from build123d import *

# Parameters (mm, degrees)
SKETCH_1_R      = 1.5
SKETCH_1_R_2    = 6.5
SKETCH_1_W      = 4
SKETCH_1_H      = 4.8
SKETCH_1_H_2    = 5
EXTRUDE_1_DEPTH = 4


with BuildPart() as part:
    # 草图1 → 凸台-拉伸1 (new body)
    with BuildSketch(Plane.XY):
        with BuildLine():
            Line((-11.37741807, 44.104762576), (9.62258193, 44.104762576))
            Line((9.62258193, 44.104762576), (17.62258193, 44.104762576))
            Line((17.62258193, 44.104762576), (38.62258193, 44.104762576))
            ThreePointArc((38.62258193, 44.104762576), (58.62258193, 24.104762576), (38.62258193, 4.104762576))
            Line((38.62258193, 4.104762576), (-11.37741807, 4.104762576))
            ThreePointArc((-11.37741807, 4.104762576), (-31.37741807, 24.104762576), (-11.37741807, 44.104762576))
        make_face()
        with Locations((1.12258193, 12.583043954)):
            Circle(SKETCH_1_R, mode=Mode.SUBTRACT)
        with Locations(Location((26.12258193, 12.583043954, 0), (0, 0, 180))):
            Circle(SKETCH_1_R, mode=Mode.SUBTRACT)
        with Locations((13.62258193, 24.104762576)):
            Circle(SKETCH_1_R, mode=Mode.SUBTRACT)
        with Locations((-11.37741807, 24.104762576)):
            Circle(SKETCH_1_R_2, mode=Mode.SUBTRACT)
        with Locations((38.62258193, 24.104762576)):
            Circle(SKETCH_1_R_2, mode=Mode.SUBTRACT)
        with Locations((29.363598717, 38.36208455)):
            Circle(SKETCH_1_R, mode=Mode.SUBTRACT)
        with Locations((-2.118434858, 38.36208455)):
            Circle(SKETCH_1_R, mode=Mode.SUBTRACT)
        with Locations((21.62258193, 37.474762576)):
            Rectangle(SKETCH_1_W, SKETCH_1_H, mode=Mode.SUBTRACT)
        with Locations((21.62258193, 28.344762576)):
            Rectangle(SKETCH_1_W, SKETCH_1_H_2, mode=Mode.SUBTRACT)
        with Locations((5.62258193, 37.474762576)):
            Rectangle(SKETCH_1_W, SKETCH_1_H, mode=Mode.SUBTRACT)
        with Locations((5.62258193, 28.344762576)):
            Rectangle(SKETCH_1_W, SKETCH_1_H_2, mode=Mode.SUBTRACT)
        with Locations((5.62258193, 19.114762576)):
            Rectangle(SKETCH_1_W, SKETCH_1_H_2, mode=Mode.SUBTRACT)
        with Locations((21.62258193, 19.114762576)):
            Rectangle(SKETCH_1_W, SKETCH_1_H_2, mode=Mode.SUBTRACT)
        with BuildLine():
            Line((11.87258193, 8.127075217), (11.87258193, 13.127075217))
            ThreePointArc((11.87258193, 13.127075217), (13.62258193, 14.877075217), (15.37258193, 13.127075217))
            Line((15.37258193, 13.127075217), (15.37258193, 8.127075217))
            ThreePointArc((15.37258193, 8.127075217), (13.62258193, 6.377075217), (11.87258193, 8.127075217))
        make_face(mode=Mode.SUBTRACT)
        with BuildLine():
            Line((15.37258193, 40.127075217), (15.37258193, 35.127075217))
            ThreePointArc((15.37258193, 35.127075217), (13.62258193, 33.377075217), (11.87258193, 35.127075217))
            Line((11.87258193, 35.127075217), (11.87258193, 40.127075217))
            ThreePointArc((11.87258193, 40.127075217), (13.62258193, 41.877075217), (15.37258193, 40.127075217))
        make_face(mode=Mode.SUBTRACT)
    extrude(amount=EXTRUDE_1_DEPTH)


solid = part.part
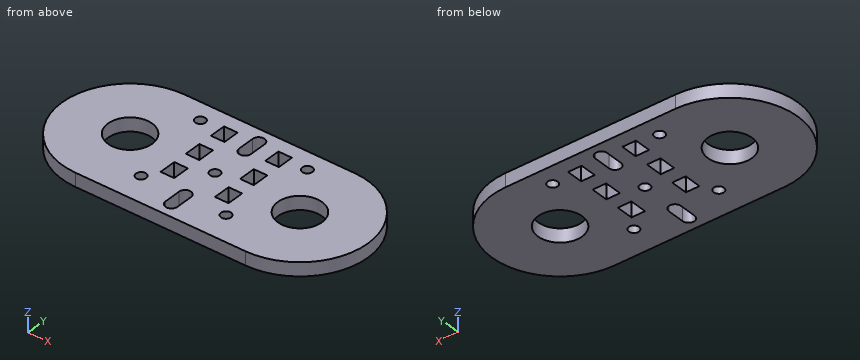
The model under review builds one solid part; all positions refer to its coordinate system, in mm. Give positions to 0.01 mm unless a question says otherwise; leave off trailing zeros. Loops run counter-clockwise (first coordinate to the right, second up) from the corner with the lowest first, then second, coordinate; pieces in that order, holes last. Notation, with made-up numbers: (13.5, 5.5) -> (49.5, 5.5) arc R35 cw to (49.5, 44.5) -> close; hole circle Ø6 at (17.25, 50.5). An arc over 180 degrees is marked (long way). Put each result on its own line as item: value. Start each with the question number.
1. We need section D-D on z = 2.45. State how many separate pieces and enclosed holes the cut face has, then the cut area to 3 significant figures.
2. Wall thickness on probe 1 along X at (y, z) = (29.5, 1.45); probe 2 along X at (y, z) = (22, 2.5); probe 3 along X at (y, z) = (22.5, 0.65): over which ranges is each line inside the solid? List them lowest first.
3. We need section C-C on y = 9. State the section outline as (x, z) points.
4. We need section A-A on x = 43.5. State the section outline as (y, z) points, then the cut area to 3 significant figures.
5. Clearance check with flat-ended pins moving along their axes: P1, Ø1, axis at y = 9.5, z = 2.5, coming from the +X side; P2, Ø2, axis at y = 19.5, z = 2.5, coming from the -X side; P3, Ø1.2, axis at y = 11.5, z = 2.5, coming from the +X side. State where each tip first meets the part, or that it passes through.
6. We need section B-B on y = 19.5. State the section outline as (x, z) points.
Determined:
1. separate pieces: 1
1. enclosed holes: 15
1. area: 2,780 mm^2
2. probe 1: -30.64 to -15, -7.75 to 3.62, 7.62 to 19.62, 23.62 to 35, 42.25 to 57.88
2. probe 2: -31.27 to -17.53, -5.23 to 32.47, 44.77 to 58.51
2. probe 3: -31.31 to -17.68, -5.08 to 32.32, 44.92 to 58.56
3. outline: (-24.49, 0) -> (11.87, 0) -> (11.87, 4) -> (-24.49, 4) -> close; (15.37, 0) -> (51.73, 0) -> (51.73, 4) -> (15.37, 4) -> close
4. outline: (4.71, 0) -> (19.81, 0) -> (19.81, 4) -> (4.71, 4) -> close; (28.4, 0) -> (43.5, 0) -> (43.5, 4) -> (28.4, 4) -> close
4. area: 121 mm^2
5. P1: x = 52.8
5. P2: x = -31.05
5. P3: x = 54.62
6. outline: (-30.84, 0) -> (-15.97, 0) -> (-15.97, 4) -> (-30.84, 4) -> close; (-6.79, 0) -> (3.62, 0) -> (3.62, 4) -> (-6.79, 4) -> close; (7.62, 0) -> (19.62, 0) -> (19.62, 4) -> (7.62, 4) -> close; (23.62, 0) -> (34.03, 0) -> (34.03, 4) -> (23.62, 4) -> close; (43.21, 0) -> (58.09, 0) -> (58.09, 4) -> (43.21, 4) -> close
